Geometry: see drawing. Coordinates: mm, zero at the bounding-box minimum. Round coordinates to 2 decimals unless told otherwise and drop trailing zeros. Loops run counter-clockwise (first coordinate to the right, second up) from the corner with the lowest first, then second, coordinate; pieces in that order, holes last. Notation, with made-up numbers: (20.25, 45) - (56.25, 45) arc R16 ccw to (56.25, 60) - close; hole circle Ø9 at (-33.5, 45.5). An arc over 180 degrees is marked (long way). Use CSV: the item, a comma, the result in double quotes.
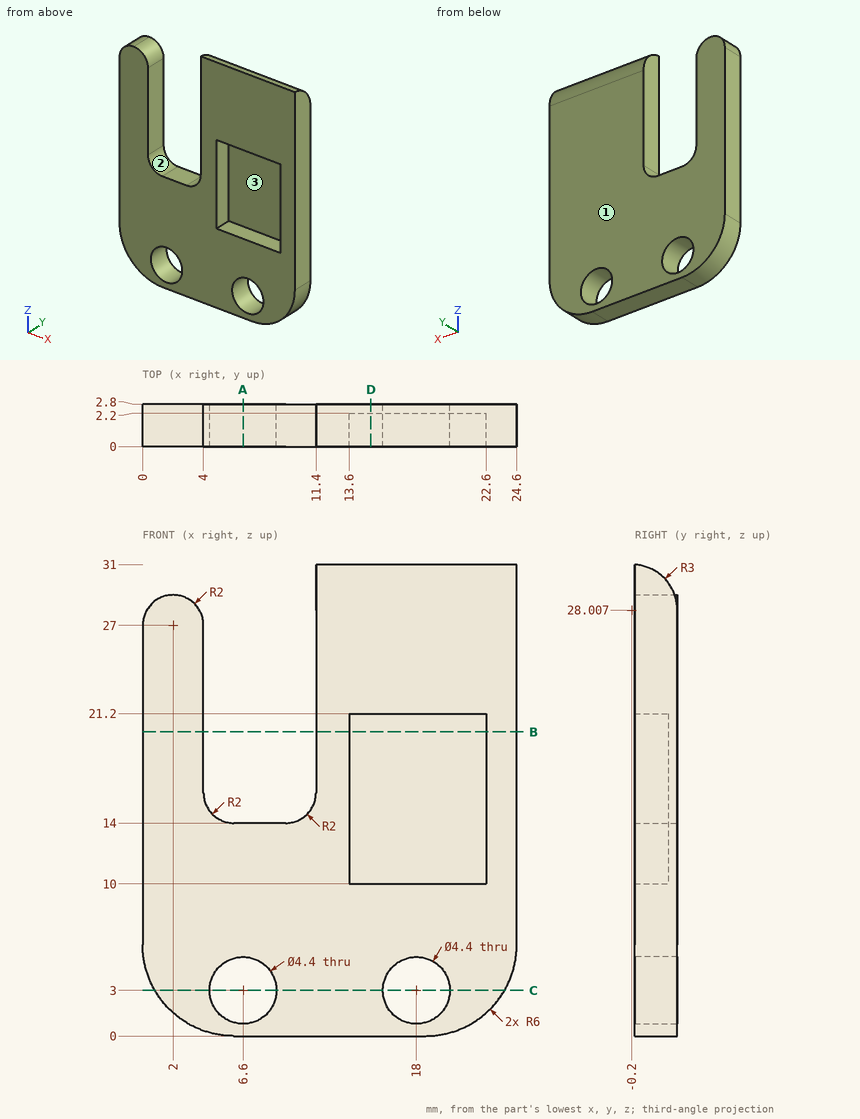
Item 1: Pin query (flat end, axial travel): P1, Ø2.5, axis at x = 19.5, z = 18, coming from the -Y side; P2, Ø0.7, axis at x = 18.5, y = 0.5, coming from the +Z side. Return the tip coordinate at first contact, or that it passes through.
Final values:
P1,"stops at y = 2.2"
P2,"stops at z = 30.99"
Item 2: Section D-D on x = 15. Return the cut outline in (y, z).
Final values:
outline,"(0, 0) - (2.8, 0) - (2.8, 28.01) arc R3 ccw to (0, 31) - (0, 21.2) - (2.2, 21.2) - (2.2, 10) - (0, 10) - close"
Item 3: Material intervals for line 1 (X direction, y = 2, z = 20); line 2 (X direction, y = 2.6, z = 25); line 3 (X direction, y = 1.3, z = 3) (1 decimal), sorted ascending.
Final values:
line 1,"x = 0 to 4, 11.4 to 13.6, 22.6 to 24.6"
line 2,"x = 0 to 4, 11.4 to 24.6"
line 3,"x = 0.8 to 4.4, 8.8 to 15.8, 20.2 to 23.8"
Item 4: Section A-A on x = 6.6. Return the cut outline in (y, z).
Final values:
outline,"(0, 0) - (2.8, 0) - (2.8, 0.8) - (0, 0.8) - close; (0, 5.2) - (2.8, 5.2) - (2.8, 14) - (0, 14) - close"
Item 5: Mould query, pull axis Z, two halves, no side actions, for the marked faces 1, 2 and 3. Classes: released by +Z, released by -Z, zero draft, split by the parting line, or undercut.
Final values:
face 1,"zero draft"
face 2,"released by +Z"
face 3,"undercut"
Item 6: Section B-B on z = 20. Return the cut outline in (x, y).
Final values:
outline,"(0, 0) - (4, 0) - (4, 2.8) - (0, 2.8) - close; (11.4, 0) - (13.6, 0) - (13.6, 2.2) - (22.6, 2.2) - (22.6, 0) - (24.6, 0) - (24.6, 2.8) - (11.4, 2.8) - close"
Item 7: Section C-C on z = 3. Return the cut outline in (x, y).
Final values:
outline,"(0.8, 0) - (4.4, 0) - (4.4, 2.8) - (0.8, 2.8) - close; (8.8, 0) - (15.8, 0) - (15.8, 2.8) - (8.8, 2.8) - close; (20.2, 0) - (23.8, 0) - (23.8, 2.8) - (20.2, 2.8) - close"
